Could you check a few things on this model? Use its own coordinates, in mm. Face numbers are marked on the shaded views. Give positions to 0.01 mm unless a question says otherwise; leave off trailing zeros. Order: outer loops, then holes, each group sorted by start corner. A loop starts at its lowest first (then second) coordinate and runs counter-clockwise, first axis right, second up. Notation, with made-up numbers: M 35.5,60 L 58.5,60 A25 cw 58.5,96 Z; hole C 12.5,-16.5 d10. An arc over 180 degrees is marked long. Use a Markdown table: item, result. Add a question column.
Item 1: If we mould it in two halves opening along X, with no side actions, what happens to the marked faces 1, 2 and 3? For each: released by +X, released by -X, zero draft, split by the parting line, or undercut.
Item 2: I'm going to push flat-ended pins straight in: pin 1 Ø3 at (y, z) = (-3, 51) entering from +X; pin 2 Ø1.5 at (x, y) = (4, -1.5) entering from -Z. Where does each tip first touch, or does it pass through?
Item 3: Suppose I cut it at A-A on x = 12.7. Write out the boundary of the cut face in (y, z) (3 decimals).
Item 4: Suppose I cut it at B-B on y = -2.25. Write out the boundary of the cut face in (x, z) (3 decimals).
Item 5: Suppose I cut it at C-C on z = 4. Write out the boundary of the cut face in (x, y), plus the area to 3 significant figures.
Item 6: If I drill on L1, parallel to Z at x = 12.7, y = -1.5 (3 decimals); L2, parallel to X at y = -4.25, z = 7; L3, parallel to Z at x = 27, y = -0.75, over which ranges is the centre line in solid material (lowest first)? Write a range as from..to.
from build123d import *

# Parameters (mm, degrees)
F0_W     = 25.4
F0_H     = 63.5
F1_DEPTH = 6.35
F2_R     = 3.175
F3_DEPTH = 6.35
F5_DEPTH = 6.35


with BuildPart() as f1:
    # F0 (on Front) → F1 (new body)
    with BuildSketch(Plane.XZ):
        with Locations((12.7, 31.75)):
            Rectangle(F0_W, F0_H)
        with BuildLine():
            Line((25.4, 0), (0, 0))
            ThreePointArc((0, 0), (12.7, -12.7), (25.4, 0))
        make_face()
    extrude(amount=F1_DEPTH)

    # F2 (on face) → F3 (cut, through all)
    with BuildSketch(Plane.XZ.offset(6.35)):
        with Locations((12.7, 0)):
            Circle(F2_R)
    extrude(amount=-F3_DEPTH, mode=Mode.SUBTRACT)

    # F4 (on face) → F5 (join, through all)
    with BuildSketch(Plane.XZ.offset(6.35)):
        with BuildLine():
            Line((25.4, 42.067379), (25.4, 41.11632))
            ThreePointArc((25.4, 41.11632), (28.170174, 43.834941), (25.4, 46.553563))
            Line((25.4, 46.553563), (25.4, 45.699533))
            ThreePointArc((25.4, 45.699533), (27.298498, 43.883456), (25.4, 42.067379))
        make_face()
    extrude(amount=-F5_DEPTH)


solid = f1.part
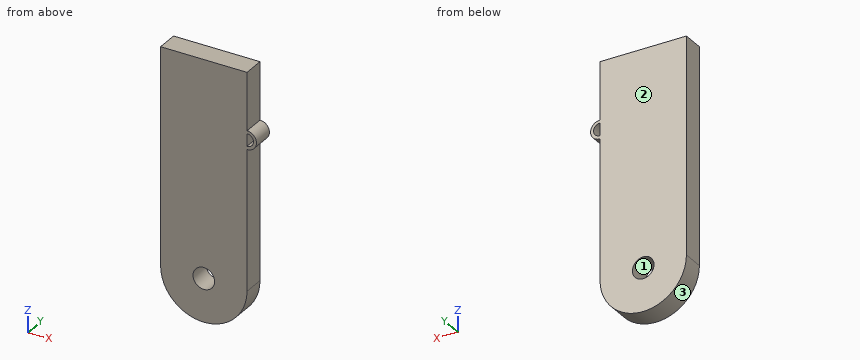
Findings below:
| question | item | result |
|---|---|---|
| 1 | face 1 | undercut |
| 1 | face 2 | zero draft |
| 1 | face 3 | split by the parting line |
| 2 | pin 1 | stops at x = 25.4 |
| 2 | pin 2 | stops at z = -9.9 |
| 3 | outline | M -6.35,-12.7 L 0,-12.7 L 0,-3.175 L -6.35,-3.175 Z; M -6.35,3.175 L 0,3.175 L 0,63.5 L -6.35,63.5 Z |
| 4 | outline | M 0,0 A12.7 ccw 25.4,0 L 25.4,41.116 A2.719 ccw long 25.4,46.554 L 25.4,63.5 L 0,63.5 Z; hole C 12.7,0 d6.35; hole M 25.4,42.067 A1.818 ccw long 25.4,45.7 Z |
| 5 | outline | M 0,-6.35 L 25.4,-6.35 L 25.4,0 L 0,0 Z |
| 5 | area | 161 mm^2 |
| 6 | L1 | z = -12.7..-3.175, 3.175..63.5 |
| 6 | L2 | x = 0..25.4 |
| 6 | L3 | z = 41.6..42.89, 44.88..46.07 |
